from build123d import *

# Parameters (mm, degrees)
SKETCH1_R           = 28.575
SKETCH1_R_2         = 12.25
SKETCH1_R_3         = 2.5908
BOSS_EXTRUDE1_DEPTH = 5
SKETCH1_3_R         = 12.25
SKETCH1_3_R_2       = 5.25
BOSS_EXTRUDE2_DEPTH = 25.4
FILLET2_R           = 0.5
SKETCH2_W           = 2
SKETCH2_H           = 1
CUT_EXTRUDE1_DEPTH  = 48.730716001
SKETCH3_R           = 2.3495
CUT_EXTRUDE4_DEPTH  = 25.4


with BuildPart() as part:
    # Sketch1 → Boss-Extrude1 (new body)
    with BuildSketch(Plane(origin=(0, 0, 0), x_dir=(1, 0, 0), z_dir=(0, 1, 0))):
        with Locations(Location((0, 0, 0), (0, 0, 270))):
            Circle(SKETCH1_R)
        with Locations(Location((0, 0, 0), (0, 0, 270))):
            Circle(SKETCH1_R_2, mode=Mode.SUBTRACT)
        with Locations(Location((-20.622229928, 11.90625, 0), (0, 0, 270))):
            Circle(SKETCH1_R_3, mode=Mode.SUBTRACT)
        with Locations(Location((-20.622229928, -11.90625, 0), (0, 0, 270))):
            Circle(SKETCH1_R_3, mode=Mode.SUBTRACT)
        with Locations(Location((0, -23.8125, 0), (0, 0, 270))):
            Circle(SKETCH1_R_3, mode=Mode.SUBTRACT)
        with Locations(Location((20.622229928, -11.90625, 0), (0, 0, 270))):
            Circle(SKETCH1_R_3, mode=Mode.SUBTRACT)
        with Locations(Location((20.622229928, 11.90625, 0), (0, 0, 270))):
            Circle(SKETCH1_R_3, mode=Mode.SUBTRACT)
        with Locations(Location((0, 23.8125, 0), (0, 0, 270))):
            Circle(SKETCH1_R_3, mode=Mode.SUBTRACT)
    extrude(amount=BOSS_EXTRUDE1_DEPTH)

    # Sketch1_3 → Boss-Extrude2 (add)
    with BuildSketch(Plane(origin=(0, 0, 0), x_dir=(1, 0, 0), z_dir=(0, 1, 0))):
        with Locations(Location((0, 0, 0), (0, 0, 270))):
            Circle(SKETCH1_3_R)
        with Locations(Location((0, 0, 0), (0, 0, 270))):
            Circle(SKETCH1_3_R_2, mode=Mode.SUBTRACT)
    extrude(amount=BOSS_EXTRUDE2_DEPTH)

    # Fillet2
    fillet2_edges = [part.edges().sort_by_distance(p)[0] for p in [
        (0, 25.4, -12.25),
        (0, 5, -28.575),
    ]]
    fillet(fillet2_edges, radius=FILLET2_R)

    # Sketch2 → Cut-Extrude1 (cut, through all)
    with BuildSketch(Plane(origin=(0, 25.4, 0), x_dir=(1, 0, 0), z_dir=(0, 1, 0))):
        with Locations((0, 5.25)):
            Rectangle(SKETCH2_W, SKETCH2_H)
    extrude(amount=-CUT_EXTRUDE1_DEPTH, mode=Mode.SUBTRACT)

    # Sketch3 → Cut-Extrude4 (cut)
    with BuildSketch(Plane.XY.offset(-5.75)):
        with Locations(Location((0, 15, 0), (0, 0, 180))):
            Circle(SKETCH3_R)
    extrude(amount=CUT_EXTRUDE4_DEPTH, mode=Mode.SUBTRACT)


solid = part.part
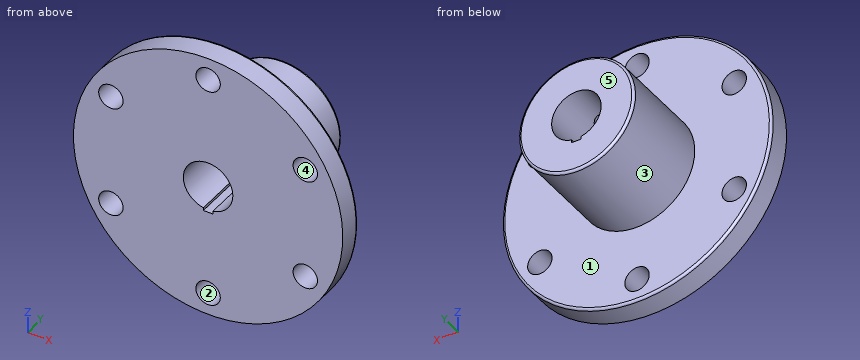
Can you work these out from the model? Positions are in its coordinate system, mm. Face numbers are marked on the shaded views. A direction names the side the tool comes from. Give positions to 0.01 mm unless a question says otherwise; leave off trailing zeros. Write each loop counter-clockwise with the first axis right and the second up, starting at its lowest first coordinate (ties: lowest second). Pieces come first, ordered by that corner, then holes. Notation, with made-up numbers: M -30,25.5 L 4,25.5 A35 ccw 4,59.5 Z; hole C -31.75,27.25 d1. An arc over 180 degrees is marked long. Answer in a Markdown table with one row per item. Add a question column.
Item 1: Imagine slicing it at B-B, the plane y = 23.5. Write out the boundary of the cut face in (x, z), plus the area to 3 significant figures.
Item 2: On a 3-axis mill with a long thin cutter (end or side, diameter ignored), from which of +Z, -Z, +X, -X, +Y, -Y can I reach the whole of each face in a straight line? I mean the marked faces 1 and 2. Say none if no direction works.
Item 3: Please list where these lines run through material, in increasing order: L1, parallel to X at y = 5.25, z = 0; L2, parallel to Y at x = 0, z = 9; L3, parallel to Y at x = -11.5, z = -16.
Item 4: We'd pull the mould along Z, two halves only. Please class the marked faces 3, 4 and 5: released by +Z, released by -Z, zero draft, split by the parting line, or undercut.
Item 5: For pin 1 Ø0.7 at (y, z) = (20.5, -5.5) entering from +X; pin 2 Ø6 at (x, y) = (-0.5, 20) entering from -Z; pin 3 Ø2.5 at (x, y) = (0.5, 18.5) entering from +Z, each with a flat end and sliding along its axis, tell me the tip position at first contact or that it passes through.
Item 6: Imagine slicing it at D-D, the plane y = 15. Write out the boundary of the cut face in (x, z).
Item 7: Imagine slicing it at A-A, the plane z = 0. Write out the boundary of the cut face in (x, y) (3 decimals), plus the area to 3 significant figures.
Item 8: Imagine slicing it at C-C, the plane x = 0. State how many separate pieces and enclosed holes the cut face has, plus the area to 3 significant figures.
Evaluation:
| question | item | result |
|---|---|---|
| 1 | outline | C 0,0 d24.5; hole M -1,-5.75 L 1,-5.75 L 1,-5.15 A5.25 ccw long -1,-5.15 Z |
| 1 | area | 384 mm² |
| 2 | face 1 | +Y |
| 2 | face 2 | +Y, -Y |
| 3 | L1 | x = -12.25 to -5.25, 5.25 to 12.25 |
| 3 | L2 | y = 0 to 12.65, 17.35 to 25.4 |
| 3 | L3 | y = 0 to 5 |
| 4 | face 3 | split by the parting line |
| 4 | face 4 | undercut |
| 4 | face 5 | zero draft |
| 5 | pin 1 | stops at x = 11.11 |
| 5 | pin 2 | stops at z = -12.25 |
| 5 | pin 3 | stops at z = 12.25 |
| 6 | outline | M -2.35,-5.75 L -2.35,-4.69 A5.25 cw -2.35,4.69 L -2.35,12.02 A12.25 ccw long 2.35,12.02 L 2.35,4.69 A5.25 cw 2.35,-4.69 L 2.35,-5.75 Z |
| 7 | outline | M -28.575,0 L -5.25,0 L -5.25,25.4 L -11.75,25.4 A0.5 ccw -12.25,24.9 L -12.25,5 L -28.075,5 A0.5 ccw -28.575,4.5 Z; M 5.25,0 L 28.575,0 L 28.575,4.5 A0.5 ccw 28.075,5 L 12.25,5 L 12.25,24.9 A0.5 ccw 11.75,25.4 L 5.25,25.4 Z |
| 7 | area | 519 mm² |
| 8 | separate pieces | 5 |
| 8 | enclosed holes | 0 |
| 8 | area | 421 mm² |
